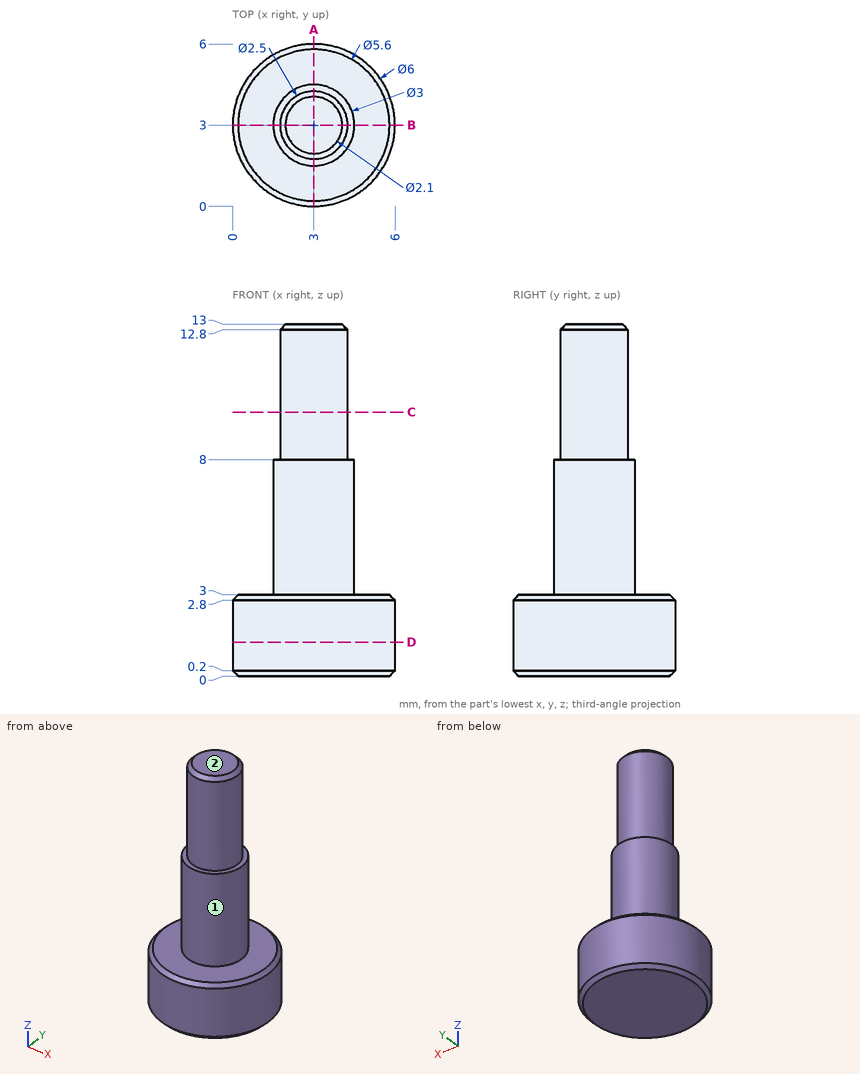
Design review of the part shown in the three views and the two pictorial views. Dimensions are in mm from the part's minimum x, y and z. A direction names the side the tool comes from. Round coordinates to 2 decimals unless told otherwise and drop trailing zeros. Loops run counter-clockwise (first coordinate to the right, second up) from the corner with the lowest first, then second, coordinate; pieces in that order, holes last. Notation, with made-up numbers: (68.5, 10.25) -> (94.5, 10.25) arc R24 cw to (94.5, 27.25) -> close; hole circle Ø9 at (15, 82.5). An arc over 180 degrees is marked (long way). Answer as CSV lines item,"result".
1) Add section A-A on x = 3. Write out the cut boundary in (y, z).
Geometry results:
outline,"(0, 0.2) -> (0.2, 0) -> (5.8, 0) -> (6, 0.2) -> (6, 2.8) -> (5.8, 3) -> (4.5, 3) -> (4.5, 8) -> (4.25, 8) -> (4.25, 12.8) -> (4.05, 13) -> (1.95, 13) -> (1.75, 12.8) -> (1.75, 8) -> (1.5, 8) -> (1.5, 3) -> (0.2, 3) -> (0, 2.8) -> close"
2) Add section D-D on z = 1.25. Write out the cut boundary in (x, y).
Geometry results:
outline,"circle Ø6 at (3, 3)"
3) To check wall thickness, follow line 1 along Z through (x, y) = (4.9, 3.8); line 2 along Z through (x, y) = (1.8, 2.2); line 3 along Y through (x, z) = (0.85, 1). State the ranges of each line that lie inside material, in increasing order. Write a range as from..to.
Geometry results:
line 1,"z = 0..3"
line 2,"z = 0..8"
line 3,"y = 0.91..5.09"
4) Add section C-C on z = 9.75. Write out the cut boundary in (x, y), plus the area to 3 significant figures.
Geometry results:
outline,"circle Ø2.5 at (3, 3)"
area,"4.91 mm²"
5) For P1, Ø2, axis at x = 4.5, y = 3, coming from the +Z side, flat-tipped, find the tip position at first contact; note if it passes through.
Geometry results:
P1,"stops at z = 13"
6) Tool access review of the marked faces 1 and 2: name each direction out of +Z, -Z, +X, -X, +Y, -Y from which nothing blocks a thin tool from reaching the whole face with its end or side.
Geometry results:
face 1,"+Z"
face 2,"+Z, +X, -X, +Y, -Y"
